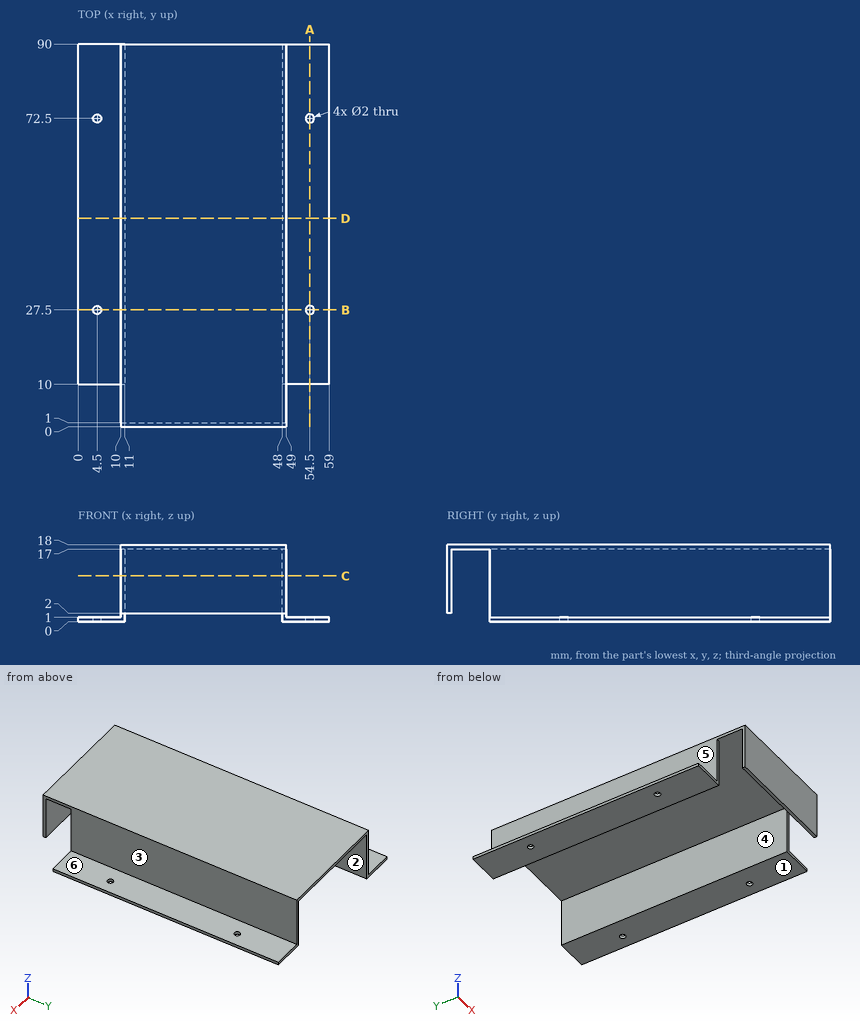
Design review of the part shown in the three views and the two pictorial views. Dimensions are in mm from the part's minimum x, y and z. A direction names the side the tool comes from. Coordinates: 2 decimals unless noted, no trailing zeros. Write each loop counter-clockwise with the first axis right and the second up, starting at its lowest first coordinate (ties: lowest second). Pieces come first, ordered by that corner, then holes.
1) Clearance check with flat-ended pins moving along their axes: pin 1 Ø2.5 at (x, y) = (54.5, 72.5) entering from +Z; pin 2 Ø8.5 at (y, z) = (65, 13) entering from +X; pin 3 Ø5 at (y, z) = (41, 8.5) entering from -X. State where each tip first meets the part, or that it passes through.
2) We need section B-B on y = 27.5. State the section outline as (x, z) points, then the cut area to 3 significant figures.
3) We need section C-C on z = 10.75. State the section outline as (x, y) points, then the cut area to 3 significant figures.
4) We need section D-D on y = 49. State the section outline as (x, z) points.
5) To check wall thickness, follow probe 1 along X at (y, z) = (72.5, 0.4); probe 2 along Y at (x, z) = (4.5, 0.3); probe 3 along X at (y, z) = (83.5, 16.75). State the ranges of each line that lie inside material, in increasing order.
6) The part is to be moulded in two halves that separate along X. For the marked faces 1, 2 and 3, say which applies: pulls with the +X half, pulls with the -X half, needs draft (parallel to the pull), parting line crosses it, or undercut.
7) We need section A-A on x = 54.5. State the section outline as (y, z) points.
8) Machinability: for the marked faces 4, 5 and 6, which of the approach directions +Z, -Z, +X, -X, +Y, -Y give a long, thin tool a straight path to every point of the face, cutting with its end or side? Answer none if there is none.
Answer list:
1. pin 1: stops at z = 1
1. pin 2: stops at x = 49
1. pin 3: stops at x = 10
2. outline: (0, 0) - (3.5, 0) - (3.5, 1) - (0, 1) - close; (5.5, 0) - (11, 0) - (11, 17) - (48, 17) - (48, 0) - (53.5, 0) - (53.5, 1) - (49, 1) - (49, 18) - (10, 18) - (10, 1) - (5.5, 1) - close; (55.5, 0) - (59, 0) - (59, 1) - (55.5, 1) - close
2. area: 89.0 mm2
3. outline: (10, 0) - (49, 0) - (49, 1) - (10, 1) - close; (10, 10) - (11, 10) - (11, 90) - (10, 90) - close; (48, 10) - (49, 10) - (49, 90) - (48, 90) - close
3. area: 199 mm2
4. outline: (0, 0) - (11, 0) - (11, 17) - (48, 17) - (48, 0) - (59, 0) - (59, 1) - (49, 1) - (49, 18) - (10, 18) - (10, 1) - (0, 1) - close
5. probe 1: x = 0 to 3.5, 5.5 to 11, 48 to 53.5, 55.5 to 59
5. probe 2: y = 10 to 26.5, 28.5 to 71.5, 73.5 to 90
5. probe 3: x = 10 to 11, 48 to 49
6. face 1: needs draft
6. face 2: undercut
6. face 3: pulls with the +X half
7. outline: (10, 0) - (26.5, 0) - (26.5, 1) - (10, 1) - close; (28.5, 0) - (71.5, 0) - (71.5, 1) - (28.5, 1) - close; (73.5, 0) - (90, 0) - (90, 1) - (73.5, 1) - close
8. face 4: -Z, +Y
8. face 5: +Z, -X, +Y, -Y
8. face 6: +Z, +X, +Y, -Y
